```python
from build123d import *

# Parameters (mm, degrees)
BOSS_EXTRU_1_DEPTH           = 0.75
ESQUISSE5_R                  = 1
R_P_TITION_CIRCULAIRE1_COUNT = 6
CONG_1_R                     = 1
CONG_3_R                     = 1
CONG_2_R                     = 0.5


with BuildPart() as part:
    # Esquisse1 → R_volution1 (revolve)
    with BuildSketch(Plane.XY, mode=Mode.PRIVATE) as r_volution1_sk:
        Polygon((0, 13.5), (0, 15), (6, 15), (7, 4), (8, 4), (8, 0), (3, 0), (3, 13.5), align=None)
    revolve(r_volution1_sk.sketch.rotate(Axis((0, 13.5, 0), (0, 1, 0)), 90), axis=Axis((0, 13.5, 0), (0, 1, 0)))

    # Esquisse2 → Boss.-Extru.1 (add, symmetric)
    with BuildSketch(Plane.XY):
        Polygon((0, 13.844024699), (0, 15.6), (-6.5, 15.6), (-7.917715453, 0.005130014), (-6.239023438, 0), (-4.974172869, 13.844024699), align=None)
    extrude(amount=BOSS_EXTRU_1_DEPTH, both=True)

    # Enl_vement de mati_re-Balayage1: sweep along a path in Esquisse4
    with BuildLine(Plane.XY) as enl_vement_de_mati_re_balayage1_path:
        Line((6, 15), (7, 4))
    # Esquisse5 → Enl_vement de mati_re-Balayage1 (sweep, cut)
    with BuildSketch(Plane(origin=(0, 15, 0), x_dir=(1, 0, 0), z_dir=(0, 1, 0))):
        with Locations((6.7, 0)):
            Circle(ESQUISSE5_R)
    enl_vement_de_mati_re_balayage1 = sweep(path=enl_vement_de_mati_re_balayage1_path.line, mode=Mode.SUBTRACT)

    # R_p_tition circulaire1: Enl_vement de mati_re-Balayage1 ×6 about axis, 1 skipped
    r_p_tition_circulaire1_axis = Axis((0, 4, 0), (0, -1, 0))
    add([enl_vement_de_mati_re_balayage1.rotate(r_p_tition_circulaire1_axis, i * 360 / R_P_TITION_CIRCULAIRE1_COUNT) for i in range(1, R_P_TITION_CIRCULAIRE1_COUNT) if i not in (3,)], mode=Mode.SUBTRACT)

    # Cong_1
    # the kernel refuses this fillet: 1 mm, written as the material it takes off along each edge
    with BuildSketch(Plane(origin=(0, 15, 0), x_dir=(-0.2529676118012608, 0, -0.9674747476702256), z_dir=(0.9674747476702256, 0, -0.2529676118012608))) as cong_1_piece_1_section:
        with BuildLine():
            CenterArc((6 - CONG_1_R * 0.913214637926, -CONG_1_R), CONG_1_R, 5.194428908, 84.805571092)
            Line((6 + CONG_1_R * 0.0826785685416, -CONG_1_R * 0.909464253957), (6, 0))
            Line((6, 0), (6 - CONG_1_R * 0.913214637926, 0))
        make_face()
    cong_1_piece_1 = revolve(axis=Axis((0, 15, 0), (0, 1, 0)), revolution_arc=89.969771407, mode=Mode.PRIVATE)
    cong_1_piece_1 = split(cong_1_piece_1, bisect_by=Plane(origin=(-4.339518373, 14.746776321, -0.75), z_dir=(0, 0, -1)), keep=Keep.TOP, mode=Mode.PRIVATE)
    add(cong_1_piece_1, mode=Mode.SUBTRACT)
    with BuildSketch(Plane(origin=(0, 15, 0), x_dir=(-0.2529676118012608, 0, -0.9674747476702256), z_dir=(0.9674747476702256, 0, -0.2529676118012608))) as cong_1_piece_2_section:
        with BuildLine():
            CenterArc((6 - CONG_1_R * 0.913214637926, -CONG_1_R), CONG_1_R, 5.194428908, 84.805571092)
            Line((6 + CONG_1_R * 0.0826785685416, -CONG_1_R * 0.909464253957), (6, 0))
            Line((6, 0), (6 - CONG_1_R * 0.913214637926, 0))
        make_face()
    cong_1_piece_2 = revolve(axis=Axis((0, 15, 0), (0, 1, 0)), revolution_arc=89.969771407, mode=Mode.PRIVATE)
    cong_1_piece_2 = split(cong_1_piece_2, bisect_by=Plane(origin=(-5.718137903, 14.786731032, 0.75), z_dir=(0, 0, 1)), keep=Keep.TOP, mode=Mode.PRIVATE)
    add(cong_1_piece_2, mode=Mode.SUBTRACT)
    with BuildSketch(Plane(origin=(0, 15, 0), x_dir=(0.2529663770173626, 0, 0.9674750705308689), z_dir=(-0.9674750705308689, 0, 0.2529663770173626))) as cong_1_piece_3:
        with BuildLine():
            CenterArc((6 - CONG_1_R * 0.913214637926, -CONG_1_R), CONG_1_R, 5.194428908, 84.805571092)
            Line((6 + CONG_1_R * 0.0826785685416, -CONG_1_R * 0.909464253957), (6, 0))
            Line((6, 0), (6 - CONG_1_R * 0.913214637926, 0))
        make_face()
    revolve(axis=Axis((0, 15, 0), (0, 1, 0)), revolution_arc=90.693766423, mode=Mode.SUBTRACT)
    with BuildSketch(Plane(origin=(0, 15, 0), x_dir=(-0.7113748000991912, 0, 0.7028128440657838), z_dir=(-0.7028128440657838, 0, -0.7113748000991912))) as cong_1_piece_4:
        with BuildLine():
            CenterArc((6 - CONG_1_R * 0.913214637926, -CONG_1_R), CONG_1_R, 5.194428908, 84.805571092)
            Line((6 + CONG_1_R * 0.0826785685416, -CONG_1_R * 0.909464253957), (6, 0))
            Line((6, 0), (6 - CONG_1_R * 0.913214637926, 0))
        make_face()
    revolve(axis=Axis((0, 15, 0), (0, 1, 0)), revolution_arc=90.693766423, mode=Mode.SUBTRACT)
    with BuildSketch(Plane(origin=(0, 15, 0), x_dir=(-0.9676080758147573, 0, -0.25245714808272485), z_dir=(0.25245714808272485, 0, -0.9676080758147573))) as cong_1_piece_5_section:
        with BuildLine():
            CenterArc((6 - CONG_1_R * 0.913214637926, -CONG_1_R), CONG_1_R, 5.194428908, 84.805571092)
            Line((6 + CONG_1_R * 0.0826785685416, -CONG_1_R * 0.909464253957), (6, 0))
            Line((6, 0), (6 - CONG_1_R * 0.913214637926, 0))
        make_face()
    cong_1_piece_5 = revolve(axis=Axis((0, 15, 0), (0, 1, 0)), revolution_arc=89.969771407, mode=Mode.PRIVATE)
    cong_1_piece_5 = split(cong_1_piece_5, bisect_by=Plane(origin=(-5.718137661, 14.786731089, -0.75), z_dir=(0, 0, -1)), keep=Keep.TOP, mode=Mode.PRIVATE)
    add(cong_1_piece_5, mode=Mode.SUBTRACT)
    with BuildSketch(Plane(origin=(0, 15, 0), x_dir=(-0.9676080758147573, 0, -0.25245714808272485), z_dir=(0.25245714808272485, 0, -0.9676080758147573))) as cong_1_piece_6_section:
        with BuildLine():
            CenterArc((6 - CONG_1_R * 0.913214637926, -CONG_1_R), CONG_1_R, 5.194428908, 84.805571092)
            Line((6 + CONG_1_R * 0.0826785685416, -CONG_1_R * 0.909464253957), (6, 0))
            Line((6, 0), (6 - CONG_1_R * 0.913214637926, 0))
        make_face()
    cong_1_piece_6 = revolve(axis=Axis((0, 15, 0), (0, 1, 0)), revolution_arc=89.969771407, mode=Mode.PRIVATE)
    cong_1_piece_6 = split(cong_1_piece_6, bisect_by=Plane(origin=(-4.339518374, 14.746776323, 0.75), z_dir=(0, 0, 1)), keep=Keep.TOP, mode=Mode.PRIVATE)
    add(cong_1_piece_6, mode=Mode.SUBTRACT)
    with BuildSketch(Plane(origin=(0, 15, 0), x_dir=(0.7113748000991921, 0, -0.7028128440657829), z_dir=(0.7028128440657829, 0, 0.7113748000991921))) as cong_1_piece_7:
        with BuildLine():
            CenterArc((6 - CONG_1_R * 0.913214637926, -CONG_1_R), CONG_1_R, 5.194428908, 84.805571092)
            Line((6 + CONG_1_R * 0.0826785685416, -CONG_1_R * 0.909464253957), (6, 0))
            Line((6, 0), (6 - CONG_1_R * 0.913214637926, 0))
        make_face()
    revolve(axis=Axis((0, 15, 0), (0, 1, 0)), revolution_arc=90.693766423, mode=Mode.SUBTRACT)
    with BuildSketch(Plane(origin=(0, 15, 0), x_dir=(0.9643411771165549, 0, 0.2646622264650878), z_dir=(-0.2646622264650878, 0, 0.9643411771165549))) as cong_1_piece_8:
        with BuildLine():
            CenterArc((6 - CONG_1_R * 0.913214637926, -CONG_1_R), CONG_1_R, 5.194428908, 84.805571092)
            Line((6 + CONG_1_R * 0.0826785685416, -CONG_1_R * 0.909464253957), (6, 0))
            Line((6, 0), (6 - CONG_1_R * 0.913214637926, 0))
        make_face()
    revolve(axis=Axis((0, 15, 0), (0, 1, 0)), revolution_arc=90.693766423, mode=Mode.SUBTRACT)

    # Cong_3
    cong_3_edges = [part.edges().sort_by_distance(p)[0] for p in [
        (-6.5, 15.6, 0),
    ]]
    fillet(cong_3_edges, radius=CONG_3_R)

    # Cong_2
    cong_2_edges = [part.edges().sort_by_distance(p)[0] for p in [
        (0, 15.3, -0.75),
        (0, 15.3, 0.75),
    ]]
    fillet(cong_2_edges, radius=CONG_2_R)


solid = part.part
```
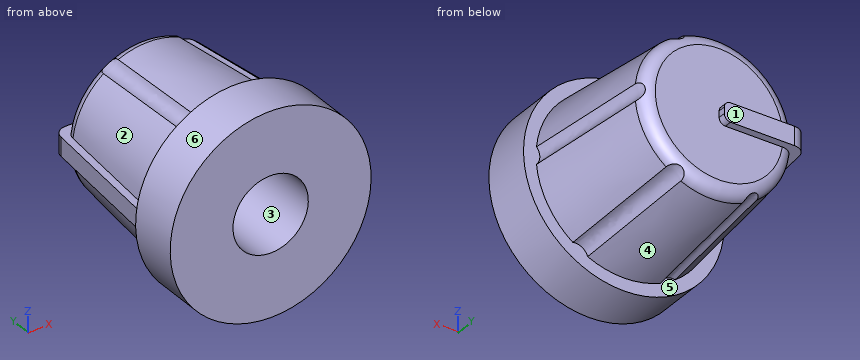
Can you work these out from the model? Positions are in its coordinate system, mm. Face numbers are marked on the shaded views. A direction names the side the tool comes from. Give positions to 0.01 mm unless a question says otherwise; leave off trailing zeros. Write item = value, one per line. Start each with the question number.
1. Thinking about a two-plate mould opening in X: for the marked faces 1, 2, 3 and 4, which applies, released by +X, released by -X, zero draft, split by the parting line, or undercut?
2. Please list where these lines run through material, in increasing order: line 1 (Y direction, x = 4, z = -2); line 2 (Y direction, x = 0, z = -2.75); line 3 (X direction, y = 5, z = 0).
3. On a 3-axis mill with a long thin cutter (end or side, diameter ignored), from which of +Z, -Z, +X, -X, +Y, -Y can I reach the whole of each face in a straight line? I mean the marked faces 5 and 6. Say none if no direction works.
4. For pin 1 (5 mm diameter, centred on x = -0.5, z = 1.5, fed in from -Y); pin 2 (5.5 mm diameter, centred on x = -2.5, y = 10.5, fed in from -Z); pin 3 (4 mm diameter, centred on x = 3, y = 14, fed in from -Z); pin 4 (8 mm diameter, centred on x = -4, y = 11.5, fed in from +Z), each with a flat end and sliding along its axis, tell me the tip position at first contact or that it passes through.
Worked answers:
q1.face_1 = zero draft
q1.face_2 = released by -X
q1.face_3 = undercut
q1.face_4 = split by the parting line
q2.line_1 = 0 to 15
q2.line_2 = 13.5 to 15
q2.line_3 = -7.46 to -3, 3 to 6.61
q3.face_5 = +Y
q3.face_6 = +Y, -Y
q4.pin_1 = 0
q4.pin_2 = -6.56
q4.pin_3 = -6.05
q4.pin_4 = 6.49
